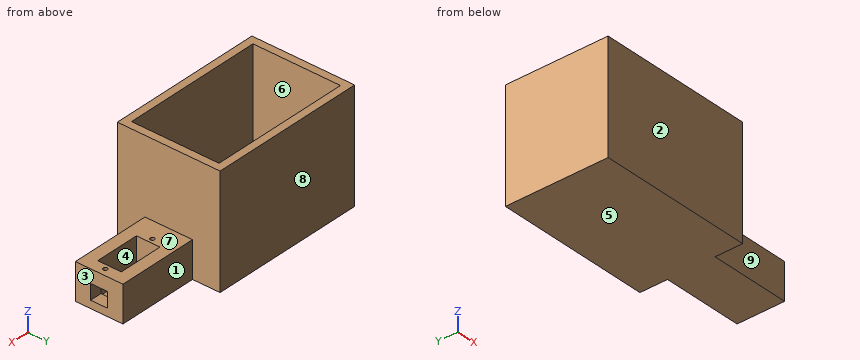
```python
from build123d import *

# Parameters (mm, degrees)
SKETCH_1_W           = 45
SKETCH_1_H           = 25
EXTRUDE_2_DEPTH      = 19
SKETCH_4_W           = 23.6
SKETCH_4_H           = 12.4
CUT_EXTRUDE_2_DEPTH  = 17.5
SKETCH_5_W           = 8
SKETCH_5_H           = 9
CUT_EXTRUDE_4_DEPTH  = 7
SKETCH_6_R           = 1.1
CUT_EXTRUDE_6_DEPTH  = 7.5
SKETCH_8_W           = 2.6
SKETCH_8_H           = 25
EXTRUDE_3_DEPTH      = 17.5
SKETCH_10_W          = 36.5
SKETCH_10_H          = 60
EXTRUDE_5_DEPTH      = 2.6
SKETCH_13_W          = 36.5
SKETCH_13_H          = 60
EXTRUDE_6_DEPTH      = 1.4
SKETCH_14_W          = 36.5
SKETCH_14_H          = 3
CUT_EXTRUDE_9_DEPTH  = 4
SKETCH_15_W          = 36.5
SKETCH_15_H          = 3
CUT_EXTRUDE_10_DEPTH = 4
SKETCH_16_W          = 4
SKETCH_16_H          = 54
EXTRUDE_7_DEPTH      = 21.5
SKETCH_17_W          = 4
SKETCH_17_H          = 54
EXTRUDE_8_DEPTH      = 78
SKETCH_18_W          = 78
SKETCH_18_H          = 4
EXTRUDE_9_DEPTH      = 54
SKETCH_19_W          = 78
SKETCH_19_H          = 4
EXTRUDE_10_DEPTH     = 54
SKETCH_20_W          = 4
SKETCH_20_H          = 46
EXTRUDE_11_DEPTH     = 54


with BuildPart() as part:
    # 草圖1 → 填料-伸長2 (new body)
    with BuildSketch(Plane.XY):
        with Locations((-42.528991691, -4.596431101)):
            Rectangle(SKETCH_1_W, SKETCH_1_H)
    extrude(amount=EXTRUDE_2_DEPTH)

    # 草圖4 → 除料-伸長2 (cut)
    with BuildSketch(Plane.XY.offset(19)):
        with Locations((-38.128991691, -4.596431101)):
            Rectangle(SKETCH_4_W, SKETCH_4_H)
    extrude(amount=-CUT_EXTRUDE_2_DEPTH, mode=Mode.SUBTRACT)

    # 草圖5 → 除料-伸長4 (cut)
    with BuildSketch(Plane(origin=(-20.028991691, 0, 0), x_dir=(0, 0, -1), z_dir=(1, 0, 0))):
        with Locations((-8, -4.596431101)):
            Rectangle(SKETCH_5_W, SKETCH_5_H)
    extrude(amount=-CUT_EXTRUDE_4_DEPTH, mode=Mode.SUBTRACT)

    # 草圖6 → 除料-伸長6 (cut)
    with BuildSketch(Plane.XY.offset(19)):
        with Locations((-23.828991691, -4.596431101)):
            Circle(SKETCH_6_R)
        with Locations((-52.428991691, -4.596431101)):
            Circle(SKETCH_6_R)
    extrude(amount=-CUT_EXTRUDE_6_DEPTH, mode=Mode.SUBTRACT)

    # 草圖8 → 填料-伸長3 (add)
    with BuildSketch(Plane.XY.offset(19)):
        with Locations((-63.728991691, -4.596431101)):
            Rectangle(SKETCH_8_W, SKETCH_8_H)
    extrude(amount=EXTRUDE_3_DEPTH)

    # 草圖10 → 填料-伸長5 (add)
    with BuildSketch(Plane(origin=(-62.428991691, 0, 0), x_dir=(0, 0, -1), z_dir=(1, 0, 0))):
        with Locations((-18.25, -4.613155897)):
            Rectangle(SKETCH_10_W, SKETCH_10_H)
    extrude(amount=-EXTRUDE_5_DEPTH)

    # 草圖13 → 填料-伸長6 (add)
    with BuildSketch(Plane.ZY.offset(65.028991691)):
        with Locations((18.25, -4.613155897)):
            Rectangle(SKETCH_13_W, SKETCH_13_H)
    extrude(amount=EXTRUDE_6_DEPTH)

    # 草圖14 → 除料-伸長9 (cut)
    with BuildSketch(Plane(origin=(-62.428991691, 0, 0), x_dir=(0, 0, -1), z_dir=(1, 0, 0))):
        with Locations((-18.25, -33.113155897)):
            Rectangle(SKETCH_14_W, SKETCH_14_H)
    extrude(amount=-CUT_EXTRUDE_9_DEPTH, mode=Mode.SUBTRACT)

    # 草圖15 → 除料-伸長10 (cut)
    with BuildSketch(Plane(origin=(-62.428991691, 0, 0), x_dir=(0, 0, -1), z_dir=(1, 0, 0))):
        with Locations((-18.25, 23.886844103)):
            Rectangle(SKETCH_15_W, SKETCH_15_H)
    extrude(amount=-CUT_EXTRUDE_10_DEPTH, mode=Mode.SUBTRACT)

    # 草圖16 → 填料-伸長7 (add)
    with BuildSketch(Plane.XY.offset(36.5)):
        with Locations((-64.428991691, -4.613155897)):
            Rectangle(SKETCH_16_W, SKETCH_16_H)
    extrude(amount=EXTRUDE_7_DEPTH)

    # 草圖17 → 填料-伸長8 (add)
    with BuildSketch(Plane.ZY.offset(66.428991691)):
        with Locations((2, -4.613155897)):
            Rectangle(SKETCH_17_W, SKETCH_17_H)
    extrude(amount=EXTRUDE_8_DEPTH)

    # 草圖18 → 填料-伸長9 (add)
    with BuildSketch(Plane.XY.offset(4)):
        with Locations((-105.428991691, 20.386844103)):
            Rectangle(SKETCH_18_W, SKETCH_18_H)
    extrude(amount=EXTRUDE_9_DEPTH)

    # 草圖19 → 填料-伸長10 (add)
    with BuildSketch(Plane.XY.offset(4)):
        with Locations((-105.428991691, -29.613155897)):
            Rectangle(SKETCH_19_W, SKETCH_19_H)
    extrude(amount=EXTRUDE_10_DEPTH)

    # 草圖20 → 填料-伸長11 (add)
    with BuildSketch(Plane.XY.offset(4)):
        with Locations((-142.428991691, -4.613155897)):
            Rectangle(SKETCH_20_W, SKETCH_20_H)
    extrude(amount=EXTRUDE_11_DEPTH)


solid = part.part
```
Design review of the part built by this model. Coordinates are the model's own, in mm. Face numbers are marked on the shaded views. A direction names the side the tool comes from. Round coordinates to 2 decimals unless told otherwise and drop trailing zeros. Order: outer loops, then holes, each group sorted by start corner. A loop starts at its lowest first (then second) coordinate and runs counter-clockwise, first axis right, second up. Notation, with made-up numbers: (15, 8) - (35, 8) arc R16 cw to (35, 18) - close; hole circle Ø5 at (-16.5, 86). An arc over 180 degrees is marked (long way). Return JSON: item names as keys, results as strings.
Q1. Wall thickness on L1, parallel to X at y = 13, z = 34.5; L2, parallel to X at y = 6, z = 13; L3, parallel to Z at x = -26, y = -8.5: over which ranges is each line inside the solid? List them lowest first. Write a range as [from, to].
Computed values:
{"L1": "x = [-144.43, -140.43], [-66.43, -62.43]", "L2": "x = [-144.43, -140.43], [-66.43, -20.03]", "L3": "z = [0, 4], [12, 19]"}
Q2. Consider section D-D on z = 45. Write out the cut boundary in (x, y), plus the area to 3 significant figures.
Computed values:
{"outline": "(-144.43, -31.61) - (-62.43, -31.61) - (-62.43, 22.39) - (-144.43, 22.39) - close; hole (-140.43, -27.61) - (-66.43, -27.61) - (-66.43, 18.39) - (-140.43, 18.39) - close", "area": "1,020 mm2"}
Q3. Machinability: for the marked faces 5, 6, 7, 8 and 9, which of the approach directions +Z, -Z, +X, -X, +Y, -Y give a long, thin tool a straight path to every point of the face, cutting with its end or side? Answer none if there is none.
Computed values:
{"face 5": "-Z, +X, -X, +Y, -Y", "face 6": "+Z", "face 7": "+Z, +X, +Y, -Y", "face 8": "+Z, -Z, +X, -X, +Y", "face 9": "+Z, -Z, +X, -Y"}
Q4. Consider section C-C on x = -120. Write out the cut boundary in (y, z), plus the area to 3 significant figures.
Computed values:
{"outline": "(-31.61, 0) - (22.39, 0) - (22.39, 58) - (18.39, 58) - (18.39, 4) - (-27.61, 4) - (-27.61, 58) - (-31.61, 58) - close", "area": "648 mm2"}
Q5. For pin 1 Ø6 at (y, z) = (-19.5, 49) entering from +X; pin 2 Ø21 at (x, z) = (-35, 5) entering from -Y; pin 3 Ø20 at (x, y) = (-49, 0.5) entering from +Z, all flat-tipped, find the tip position at first contact; note any pin that passes through.
Computed values:
{"pin 1": "stops at x = -62.43", "pin 2": "stops at y = -17.1", "pin 3": "stops at z = 19"}
Q6. The part is to be moulded in two halves that separate along Y. For the marked faces 1, 2, 3 and 4, say which applies: pulls with the +Y half, pulls with the -Y half, needs draft (parallel to the pull), parting line crosses it, or undercut.
Computed values:
{"face 1": "pulls with the +Y half", "face 2": "pulls with the -Y half", "face 3": "needs draft", "face 4": "undercut"}
Q7. Consider section B-B on y = -22. Write out the cut boundary in (x, z), plus the area to 3 significant figures.
Computed values:
{"outline": "(-144.43, 0) - (-62.43, 0) - (-62.43, 58) - (-66.43, 58) - (-66.43, 4) - (-140.43, 4) - (-140.43, 58) - (-144.43, 58) - close", "area": "760 mm2"}
Q8. Consider section A-A on z = 9. Write out the cut boundary in (x, y).
Computed values:
{"outline": "(-144.43, -31.61) - (-62.43, -31.61) - (-62.43, -17.1) - (-20.03, -17.1) - (-20.03, -9.1) - (-26.33, -9.1) - (-26.33, -10.8) - (-49.93, -10.8) - (-49.93, 1.6) - (-26.33, 1.6) - (-26.33, -0.1) - (-20.03, -0.1) - (-20.03, 7.9) - (-62.43, 7.9) - (-62.43, 22.39) - (-144.43, 22.39) - close; hole (-140.43, -27.61) - (-66.43, -27.61) - (-66.43, 18.39) - (-140.43, 18.39) - close"}
